Autodesk Inventor part; units mm, degrees
ref_plane "Work Plane1" through (-20, 0, 0) normal (0, 1, 0) x (1, 0, 0)
ref_plane "YZ Plane" through (0, 0, 0) normal (1, 0, 0) x (0, 1, 0)
ref_plane "XZ Plane" through (0, 0, 0) normal (0, 1, 0) x (-1, 0, 0)
sketch "Sketch1" plane through (0, 0, 0) normal (0, 0, 1) x (1, 0, 0)
  line L0 (-20, -20) -> (20, -20)
  line L1 (20, -20) -> (20, 20)
  line L2 (20, 20) -> (-20, 20)
  line L3 (-20, 20) -> (-20, -20)
  line L4 (-20, -20) -> (20, 20) construction
  line L5 (20, -20) -> (-20, 20) construction
  point P0 (0, 0)
  dimension "d0" = 40
  dimension "d1" = 40
extrude "Extrusion1" add sketch "Sketch1" along normal blind 10
sketch "Sketch2" plane through (0, 0, 10) normal (0, 0, 1) x (1, 0, 0)
  circle A0 centre (0, 0) radius 19
  line L0 (-10.247, 16) -> (10.247, 16)
  line L1 (-13.8564, 13) -> (13.8564, 13)
  line L2 (-16.1555, 10) -> (16.1555, 10)
  line L3 (-17.6635, 7) -> (17.6635, 7)
  line L4 (-18.5742, 4) -> (18.5742, 4)
  circle A1 centre (0, 16) radius 2.38
  circle A2 centre (-6.5, 13) radius 2.38
  circle A3 centre (6.5, 13) radius 2.38
  circle A4 centre (-12, 10) radius 2.38
  circle A5 centre (0, 10) radius 2.38
  circle A6 centre (12, 10) radius 2.38
  circle A7 centre (-6.5, 7) radius 2.38
  circle A8 centre (6.5, 7) radius 2.38
  circle A9 centre (-14, 4) radius 2.38
  circle A10 centre (0, 4) radius 2.38
  circle A11 centre (14, 4) radius 2.38
  circle A12 centre (-7, 0) radius 2.38
  circle A13 centre (7, 0) radius 2.38
  dimension "d4" = 38
  dimension "d5" = 4.76
  dimension "d6" = 4.76
  dimension "d7" = 4.76
  dimension "d8" = 3
  dimension "d9" = 3
  dimension "d10" = 16
  dimension "d11" = 6.5
  dimension "d12" = 6.5
  dimension "d13" = 12
  dimension "d14" = 12
  dimension "d15" = 3
  dimension "d16" = 3
  dimension "d17" = 14
  dimension "d18" = 14
  dimension "d19" = 7
  dimension "d20" = 7
extrude "Extrusion2" cut sketch "Sketch2" against normal up to next contours A11 L4 | L4 A11 | A9 L4 | L4 A9 | A8 L3 | L3 A8 | A7 L3 | L3 A7 | A6 L2 | L2 A6 | A10 L4 | L4 A10 | A4 L2 | L2 A4 | A3 L1 | L1 A3 | A2 L1 | L1 A2 | A1 L0 | L0 A1 | A5 L2 | L2 A5 | A12 | A13
ref_plane "Work Plane1" through (-20, 0, 0) normal (0, 1, 0) x (1, 0, 0)
mirror "Mirror1" about plane through (-20, 0, 0) normal (0, 1, 0) of "Extrusion2"
properties part number "FanTemplate40mm"
The listing builds one solid part. Answer for the finished solid, in the listing's coordinates (mm). Round coordinates to 2 decimals unless told otherwise and drop trailing zeros. Loops run counter-clockwise (first coordinate to the right, second up) from the corner with the lowest first, then second, coordinate; pieces in that order, holes last. Notation, with made-up numbers: (85.5, -4.75) -> (104.5, -4.75) arc R14 cw to (104.5, 0.25) -> close; hole circle Ø1 at (49, 60.5). An arc over 180 degrees is marked (long way). Use one line per item in the form item = value.
1. The part is cut by section C-C on z = 4.5. Give the number of separate pieces and of enclosed holes in the cut face, and give its area (3 significant figures).
Answer key:
separate_pieces = 1
enclosed_holes = 24
area = 1,170 mm²
2. The part is cut by section D-D on x = 7. Determine the outline of the cut face in (y, z).
Answer key:
outline = (-20, 0) -> (-15.33, 0) -> (-15.33, 10) -> (-20, 10) -> close; (-10.67, 0) -> (-9.33, 0) -> (-9.33, 10) -> (-10.67, 10) -> close; (-4.67, 0) -> (-2.38, 0) -> (-2.38, 10) -> (-4.67, 10) -> close; (2.38, 0) -> (4.67, 0) -> (4.67, 10) -> (2.38, 10) -> close; (9.33, 0) -> (10.67, 0) -> (10.67, 10) -> (9.33, 10) -> close; (15.33, 0) -> (20, 0) -> (20, 10) -> (15.33, 10) -> close
3. The part is cut by section B-B on y = -16. Determine the outline of the cut face in (x, z), and give its area (3 significant figures).
Answer key:
outline = (-20, 0) -> (-2.38, 0) -> (-2.38, 10) -> (-20, 10) -> close; (2.38, 0) -> (20, 0) -> (20, 10) -> (2.38, 10) -> close
area = 352 mm²
4. Find the intervals of material crossed by probe 1 along X at (y, z) = (13, 5.5); probe 2 along X at (y, z) = (4, 4.5); probe 3 along Y at (x, z) = (14.5, 4.25), in increasing order. Write a range as [from, to].
Answer key:
probe_1 = [-20, -8.88], [-4.12, 4.12], [8.88, 20]
probe_2 = [-20, -16.38], [-11.62, -2.38], [2.38, 11.62], [16.38, 20]
probe_3 = [-20, -6.33], [-1.67, 1.67], [6.33, 20]
5. The part is cut by section A-A on y = 0. Determine the outline of the cut face in (x, z).
Answer key:
outline = (-20, 0) -> (-9.38, 0) -> (-9.38, 10) -> (-20, 10) -> close; (-4.62, 0) -> (4.62, 0) -> (4.62, 10) -> (-4.62, 10) -> close; (9.38, 0) -> (20, 0) -> (20, 10) -> (9.38, 10) -> close
6. A flat-ended cylindrical pin translates along its axis: pin 1 Ø5.5 at (x, y) = (-14, 4) entering from -Z. Find the tip coordinate at first contact, or state that the pin passes through.
Answer key:
pin_1 = 0
7. For a pull along Y with two mould halves and no side action, classify faces 1 (the cylindrical face through (-5.4, 10.89, 5.07)), 2 (the flat face through (-20, 0, 5)) as released by +Y, released by -Y, zero draft, split by the parting line, or undercut.
Answer key:
face_1 = undercut
face_2 = zero draft
